Build history of the part. All positions in model axes, mm. A direction names the side the tool comes from. Coordinates: 2 decimals unless noted, no trailing zeros. Order: outer loops, then holes, each group sorted by start corner. A loop starts at its lowest first (then second) coordinate and runs counter-clockwise, first axis right, second up. Notation, with made-up numbers: (65.25, -31) -> (87.25, -31) arc R23 cw to (87.25, -5) -> close; hole circle Ø9 at (-13, 30.5). An arc over 180 degrees is marked (long way). Write each question's results on one line, items separated by ' | '.
Autodesk Inventor part; units mm, degrees
ref_plane "YZ Plane" through (0, 0, 0) normal (1, 0, 0) x (0, 1, 0)
ref_plane "XZ Plane" through (0, 0, 0) normal (0, 1, 0) x (-1, 0, 0)
ref_plane "XY Plane" through (0, 0, 0) normal (0, 0, 1) x (1, 0, 0)
sketch "Skizze1" plane through (0, 0, 0) normal (0, 0, 1) x (1, 0, 0)
  circle A0 centre (12.0667, -17.5) radius 2
  circle A1 centre (12.0667, 17.5) radius 2
  line L0 (17.0667, 22.5) -> (17.0667, -22.5)
  line L1 (7.0667, 22.5) -> (17.0667, 22.5)
  line L2 (7.0667, -22.5) -> (7.0667, 22.5)
  line L3 (17.0667, -22.5) -> (7.0667, -22.5)
  circle A2 centre (-23.4333, -17.5) radius 2
  circle A3 centre (-23.4333, 17.5) radius 2
  line L4 (-19.9333, 22.5) -> (-19.9333, -22.5)
  line L5 (-26.9333, 22.5) -> (-19.9333, 22.5)
  line L6 (-26.9333, -22.5) -> (-26.9333, 22.5)
  line L7 (-19.9333, -22.5) -> (-26.9333, -22.5)
  line L8 (43.2163, 19.557) -> (43.2163, 16.9277)
  line L9 (43.2163, -19.557) -> (43.2163, -16.9277)
  line L10 (43.2163, -20.3) -> (43.2163, -16.7)
  line L11 (43.2163, 20.3) -> (43.2163, 16.7)
  line L12 (-26.9333, 22.5) -> (43.2163, 22.5)
  line L13 (43.2163, 22.5) -> (43.2163, -22.5)
  line L14 (43.2163, -22.5) -> (-26.9333, -22.5)
  line L15 (-26.9333, -22.5) -> (-26.9333, 22.5)
  point P0 (0, 0)
extrude "Extrusion1" add sketch "Skizze1" along normal blind 5 contours A0 | A1 | L12 L13 L11 L8 L10 L9 L14 L0 | L0 L3 L2 L1 | L2 L14 L4 L12 | L4 L7 L6 L5 | A2 | A3
sketch "Skizze2" plane through (43.2163, -22.5, 0) normal (1, 0, 0) x (0, 0, -1)
  line L0 (0, 0) -> (-5, 0)
  line L1 (0, 0) -> (81.01, 0)
  line L2 (81.01, 0) -> (81.01, 45)
  line L3 (81.01, 45) -> (0, 45)
  line L4 (0, 45) -> (0, 0)
  circle A0 centre (77.01, 41) radius 1.8 construction
  circle A1 centre (77.01, 4) radius 1.8 construction
  arc A2 (54.796, 42.057) -> (57.124, 42.057) centre (55.96, 41) ccw construction
  arc A3 (57.124, 2.943) -> (54.796, 2.943) centre (55.96, 4) ccw construction
  circle A4 centre (55.96, 41) radius 1.75
  circle A5 centre (55.96, 4) radius 1.75
  circle A6 centre (77.01, 41) radius 1.75
  circle A7 centre (77.01, 4) radius 1.75
  point P0 (0, 22.5)
  dimension "d2" = 4
  dimension "d5" = 3.5
  dimension "d6" = 3.5
  dimension "d7" = 3.5
  dimension "d8" = 3.5
extrude "Extrusion2" add sketch "Skizze2" against normal blind 5
sketch "Skizze3" plane through (-26.9333, -22.5, 5) normal (0, -1, 0) x (1, 0, 0)
  line L0 (0, -5) -> (65.1497, -5)
  line L1 (31.7157, -5) -> (77.2703, -5) construction
  line L2 (65.1497, -86.01) -> (65.1497, -5)
  line L3 (51.1497, -5) -> (65.1497, -29.2487)
  line L4 (51.1497, -5) -> (79.1497, -5) construction
  line L5 (46.5308, -5) -> (65.1497, -37.2487)
  point P0 (26.9333, -5)
  dimension "d11" = 60
  dimension "d12" = 14
  dimension "d13" = 4
extrude "Extrusion3" add sketch "Skizze3" against normal up to surface (45 mm away) contours L0 L3 L2 L5
chamfer "Fasen1" distance 2 angle 45 2 edges at (38.2163, 0, 0) (43.2163, 0, 5)
sketch "Skizze4" plane through (0, 0, 5) normal (0, 0, 1) x (1, 0, 0)
  circle A0 centre (12.0667, 17.5) radius 2
  circle A1 centre (12.0667, -17.5) radius 2
  circle A2 centre (-23.4333, -17.5) radius 2
  circle A3 centre (-23.4333, 17.5) radius 2
  point P0 (0, 0)
hole "Bohrung1" at (12.0667, 17.5, 5) at (12.0667, -17.5, 5) at (-23.4333, -17.5, 5) at (-23.4333, 17.5, 5) direction (0, 0, -1) diameter 3.4 depth 8 countersink diameter 7.5 countersink angle 90
properties part number "Kameraturm_Cognex_Halter"
Item 1: Pull direction X, two halves, no side cores. Call faces 3 (the flat face through (38.216, 0, -56)), 4 (the cylindrical face through (13.575, 16.716, 1.454)), 5 (the flat face through (-4, 0, 0)): released by +X, released by -X, zero draft, split by the parting line, or undercut.
Answer:
face 3: released by -X | face 4: undercut | face 5: zero draft
Item 2: Slice it at C-C, the plane x = 35. List the corners of the cut face in (y, z), and give its area (3 significant figures).
Answer:
outline: (-22.5, -26.68) -> (22.5, -26.68) -> (22.5, -18.68) -> (-22.5, -18.68) -> close; (-22.5, 0) -> (22.5, 0) -> (22.5, 5) -> (-22.5, 5) -> close | area: 585 mm^2
Item 3: Slice it at D-D, the plane x = 0. List the corners of the cut face in (y, z), and give its area (3 significant figures).
Answer:
outline: (-22.5, 0) -> (22.5, 0) -> (22.5, 5) -> (-22.5, 5) -> close | area: 225 mm^2
Item 4: Slice it at B-B, the plane z = -77.01. List the corners of the cut face in (x, y), and give its area (3 significant figures).
Answer:
outline: (38.22, -22.5) -> (43.22, -22.5) -> (43.22, -20.25) -> (38.22, -20.25) -> close; (38.22, -16.75) -> (43.22, -16.75) -> (43.22, 16.75) -> (38.22, 16.75) -> close; (38.22, 20.25) -> (43.22, 20.25) -> (43.22, 22.5) -> (38.22, 22.5) -> close | area: 190 mm^2
Item 5: Pin check, flat tips, straight feed: pin 1 (5 mm diameter, centred on x = 5, y = 10.5, fed in from -Z); pin 2 (5.5 mm diameter, centred on y = -18.5, z = -55.96, fed in from -X); pin 3 (4.5 mm diameter, centred on x = 12.07, y = 17.5, fed in from +Z). Stop position of each tip, or through.
Answer:
pin 1: stops at z = 0 | pin 2: stops at x = 38.22 | pin 3: stops at z = 3.5
Item 6: Slice it at A-A, the plane y = -9. List the corners of the cut face in (x, z).
Answer:
outline: (-26.93, 0) -> (19.6, 0) -> (38.22, -32.25) -> (38.22, -81.01) -> (43.22, -81.01) -> (43.22, 3) -> (41.22, 5) -> (-26.93, 5) -> close; hole (24.22, 0) -> (38.22, -24.25) -> (38.22, -2) -> (36.22, 0) -> close
Item 7: Tool access for faces 1 (the conical face through (-21.89, 16.52, 3.08)), 2 (the flat face through (38.216, 0, -13)): list every direction of +Z, -Z, +X, -X, +Y, -Y with a clear straight run to the whole face (end or side of a thin tool).
Answer:
face 1: +Z | face 2: +Y, -Y
Item 8: Drill centre lines: line 1 (Y direction, x = 40.2, z = -55.96); line 2 (X direction, y = 17, z = 2); line 3 (X direction, y = 17.5, z = 1.3). Where is each one in solid material? Low to high. Write a range as from..to.
Answer:
line 1: y = -22.5..-20.25, -16.75..16.75, 20.25..22.5 | line 2: x = -26.93..-25.06, -21.81..10.44, 13.69..43.22 | line 3: x = -26.93..-25.13, -21.73..10.37, 13.77..43.22
